Autodesk Inventor part; units mm, degrees
ref_plane "YZ Plane" through (0, 0, 0) normal (1, 0, 0) x (0, 1, 0)
ref_plane "XZ Plane" through (0, 0, 0) normal (0, 1, 0) x (-1, 0, 0)
ref_plane "XY Plane" through (0, 0, 0) normal (0, 0, 1) x (1, 0, 0)
sketch "Sketch1" plane through (0, 0, 0) normal (0, 0, 1) x (1, 0, 0)
  circle A0 centre (0, 0) radius 38.1
  dimension "d2" = 76.2
extrude "Extrusion1" add sketch "Sketch1" along normal mid plane 6.35
sketch "Sketch2" plane through (0, 0, 3.175) normal (0, 0, 1) x (1, 0, 0)
  circle A0 centre (0, 0) radius 38.1
  point P0 (0, 28.575)
  dimension "d3" = 0
  dimension "d4" = 28.575
hole "Mounting Hole" at (0, 28.575, 3.175) direction (0, 0, -1) diameter 6.35 end through all
pattern_circular "Circular Pattern1" count 4 over 360 about axis through (0, 0, 0) along (0, 0, 1) of "Mounting Hole"
sketch "Sketch3" plane through (0, 0, 3.175) normal (0, 0, 1) x (1, 0, 0)
  circle A0 centre (0, 0) radius 38.1
  circle A1 centre (0, 0) radius 15.875
  dimension "d15" = 31.75
extrude "Extrusion2" add sketch "Sketch3" along normal blind 12.7 contours A1
sketch "Sketch8" plane through (0, 0, 15.875) normal (0, 0, 1) x (1, 0, 0)
  circle A0 centre (0, 0) radius 15.875
hole "Hole3" at (0, 0, 15.875) direction (0, 0, -1) diameter 16.2 depth 14.986
sketch "Sketch4" plane through (0, 0, 15.875) normal (0, 0, 1) x (1, 0, 0)
  arc A0 (-3.0359, 9.528) -> (-6.5275, 7.5757) centre (0, 0) ccw
  circle A1 centre (0, 0) radius 15.875
  line L0 (0, 0) -> (-5, 8.6603) construction
  line L1 (0, 0) -> (-10.16, 0) construction
  line L2 (-2.058, 7.8342) -> (-3.0359, 9.528)
  line L3 (-5.5564, 5.8937) -> (-6.5275, 7.5757)
  arc A2 (-2.058, 7.8342) -> (-5.5564, 5.8937) centre (0, 0) ccw
  circle A3 centre (0, 0) radius 8.1
  dimension "d46" = 60
  dimension "d47" = 4
  dimension "d48" = 20
extrude "Extrusion3" cut sketch "Sketch4" against normal up to surface (14.986 mm away) contours L2 A2 L3 A0
pattern_circular "Circular Pattern2" count 6 over 360 about axis through (0, 0, 0) along (0, 0, 1) of "Extrusion3"
fillet "Fillet1" radius 0.508 1 edges at (-15.875, 0, 3.175)
sketch "Sketch9" plane through (0, 0, -3.175) normal (0, 0, -1) x (-1, 0, 0)
  circle A0 centre (0, 0) radius 38.1
  circle A1 centre (0, 0) radius 4.7625
  dimension "d56" = 9.525
extrude "Extrusion6" cut sketch "Sketch9" against normal blind 25.4 contours A1
properties part number "Denso-6" material "ABS Plastic"
Geometry check sheet. Reference: the model listing, model coordinates, mm. A direction names the side the tool comes from. Coordinates: 2 decimals unless noted, no trailing zeros. Loops run counter-clockwise (first coordinate to the right, second up) from the corner with the lowest first, then second, coordinate; pieces in that order, holes last. Notation, with made-up numbers: (45, 63) - (81, 63) arc R17 ccw to (81, 95) - close; hole circle Ø6 at (11, 77.5). An arc over 180 degrees is marked (long way). One line per item, written item: value. Start each with the question number.
(1) Material ranges on line 1 (Z direction, x = 10.5, y = -31.5) (3 decimals); line 2 (X direction, y = 30.5, z = 1); line 3 (X direction, y = -4.5, z = 10.25), recorded low to high. Write a range as [from, to].
(2) Cross-section at D-D on x = -28. Enter the section's corners in (y, z) (1 decimal).
(3) Cross-section at A-A on x = 0. Count the separate pieces of the cut face and the enclosed holes in it, plus the area to 3 significant figures.
(4) Mould release check, pull along Y, two halves, no side actions. Record for faces 3 (the flat face through (16, -8, 3.175)), 4 (the cylindrical face through (-1.932, -31.095, -0.044)): released by +Y, released by -Y, zero draft, split by the parting line, or undercut.
(5) Tool access check on faces 1 (the cylindrical face through (31.095, -1.932, -0.044)), 2 (the flat face through (-6.238, -6.534, 8.487)). Record the directions out of +Z, -Z, +X, -X, +Y, -Y that give a thin tool (end or side, any length) a straight path to the whole face; none if there is none.
(6) Depth check by flat-ended pin: P1, Ø8.5, axis at x = 0, y = 28.575, coming from the +Z side (3 decimals); P2, Ø2, axis at x = -15, z = 2.5, coming from the -Y side; P3, Ø1.6, axis at x = -9, z = 9.5, coming from the +Y side; P4, Ø15, axis at x = 0, y = 0, coming from the -Z side (3 decimals). Enter the tip coordinate at first touch or a pass-through.
Results below:
1. line 1: z = [-3.175, 3.175]
1. line 2: x = [-22.83, -2.52], [2.52, 22.83]
1. line 3: x = [-15.22, -6.73], [6.73, 15.22]
2. outline: (-25.8, -3.2) - (-3.1, -3.2) - (-3.1, 3.2) - (-25.8, 3.2) - close; (3.1, -3.2) - (25.8, -3.2) - (25.8, 3.2) - (3.1, 3.2) - close
3. separate pieces: 4
3. enclosed holes: 0
3. area: 525 mm2
4. face 3: zero draft
4. face 4: undercut
5. face 1: +Z, -Z
5. face 2: +Z
6. P1: stops at z = 3.175
6. P2: stops at y = -35.43
6. P3: stops at y = 13.59
6. P4: stops at z = -3.175
